The model under review builds one solid part; all positions refer to its coordinate system, in mm. A direction names the side the tool comes from. Give positions to 0.01 mm unless a question says otherwise; leave off trailing zeros. Loops run counter-clockwise (first coordinate to the right, second up) from the corner with the lowest first, then second, coordinate; pieces in that order, holes last. Notation, with made-up numbers: (9.5, -13.5) -> (17.5, -13.5) arc R15 ccw to (17.5, 9.5) -> close; hole circle Ø9 at (74.25, 60.5). An arc over 180 degrees is marked (long way). Write each question's results on one line, items separated by ' | '. Start each with the question number.
Q1. We need section C-C (x = -1). Write out the cut boundary in (y, z).
Q2. Wall thickness on L1, parallel to Z at x = 11, y = -2.7; L2, parallel to Y at x = 21.15, z = -9.9; L3, parallel to X at y = -1.25, z = -0.75: over which ranges is each line inside the solid? List them lowest first. Write a range as [from, to].
Q3. We need section A-A (y = -15.75). Write out the cut boundary in (x, z), plus the area to 3 significant figures.
Q4. Insertion check: pin 1 Ø15 at (x, y) = (2, -14.5) entering from +Z; pin 2 Ø8 at (x, z) = (-7, -0.5) entering from -Y; pin 3 Ø1.2 at (y, z) = (-1.5, -3) entering from +X; pin 4 Ø1.2 at (y, z) = (-2, -2) entering from -X. Each pin has a flat end and moves straight along its axis. Give the tip position at first contact, or say it passes through.
Q5. Mouldability with a two-part tool opening along Z and no side actions: class faces 4 (the face through (-23, -28, -10)), 5 (the face through (-12.5, -1.97, 0.07)), 6 (the face through (9.5, -1.97, 0.07)), 7 (the face through (2, -28, -8)) as released by +Z, released by -Z, zero draft, split by the parting line, or undercut.
Q6. We need section D-D (x = 11). Write out the cut boundary in (y, z).
Q7. Machinability: for faces 1 (the face through (6.707, -4.063, -9.972)), 2 (the face through (-19, -2, -2)), 3 (the face through (19, -2, -2)), which of the approach directions +Z, -Z, +X, -X, +Y, -Y give a long, thin tool a straight path to every point of the face, cutting with its end or side? Answer none if there is none.
Q8. We need section B-B (z = -9). Write out the cut boundary in (x, y).
from build123d import *

# Parameters (mm, degrees)
SKETCH_R             = 1.5
PAD_DEPTH            = 4
SKETCH001_R          = 0.5
PAD001_DEPTH         = 4
FILLET_R             = 4
CHAMFER_SIZE         = 4
BODY_PLACEMENT_ANGLE = 90


with BuildPart() as part:
    # Sketch → Pad (new body)
    with BuildSketch(Plane.XY):
        Polygon((-15, 4), (15, 4), (19, 0), (19, -8), (-19, -8), (-19, 0), align=None)
        with Locations((-11, 0)):
            Circle(SKETCH_R, mode=Mode.SUBTRACT)
        with Locations((11, 0)):
            Circle(SKETCH_R, mode=Mode.SUBTRACT)
    extrude(amount=PAD_DEPTH)

    # Sketch001 (on Face2 of Pad) → Pad001 (join)
    with BuildSketch(Plane.XZ.offset(8)):
        Polygon((-25, 30), (25, 30), (25, 0), (0, 0), (-25, 0), align=None)
        with Locations((-21.15, 24.5)):
            Circle(SKETCH001_R, mode=Mode.SUBTRACT)
        with Locations((-21.15, 7)):
            Circle(SKETCH001_R, mode=Mode.SUBTRACT)
        with Locations((21.15, 7)):
            Circle(SKETCH001_R, mode=Mode.SUBTRACT)
        with Locations((21.15, 24.5)):
            Circle(SKETCH001_R, mode=Mode.SUBTRACT)
        with BuildLine():
            ThreePointArc((-16.184193, 23.938422), (-21.85, 15.75), (-16.184193, 7.561578))
            Line((-16.184193, 7.561578), (-7.409917, 4.256721))
            ThreePointArc((-7.409917, 4.256721), (-6.716549, 4.064704), (-6, 4))
            Line((-6, 4), (0, 4))
            Line((6, 4), (0, 4))
            ThreePointArc((6, 4), (6.716549, 4.064704), (7.409917, 4.256721))
            Line((7.409917, 4.256721), (16.184193, 7.561578))
            ThreePointArc((16.184193, 7.561578), (21.85, 15.75), (16.184193, 23.938422))
            Line((16.184193, 23.938422), (7.409917, 27.243279))
            ThreePointArc((7.409917, 27.243279), (6.716549, 27.435296), (6, 27.5))
            Line((0, 27.5), (6, 27.5))
            Line((-6, 27.5), (0, 27.5))
            ThreePointArc((-6, 27.5), (-6.716549, 27.435296), (-7.409917, 27.243279))
            Line((-16.184193, 23.938422), (-7.409917, 27.243279))
        make_face(mode=Mode.SUBTRACT)
    extrude(amount=PAD001_DEPTH)

    # Fillet
    fillet_edges = [part.edges().sort_by_distance(p)[0] for p in [
        (19, -8, 2),
        (-19, -8, 2),
    ]]
    fillet(fillet_edges, radius=FILLET_R)

    # Chamfer
    chamfer_edges = [part.edges().sort_by_distance(p)[0] for p in [
        (-25, -10, 30),
        (25, -10, 30),
    ]]
    chamfer(chamfer_edges, length=CHAMFER_SIZE)


with BuildPart() as part_1:
    # Body placement: moved
    add(part.part.rotate(Axis((0, 0, 0), (1, 0, 0)), BODY_PLACEMENT_ANGLE))


solid = part_1.part
Output:
1) outline: (-30, -12) -> (-27.5, -12) -> (-27.5, -8) -> (-30, -8) -> close; (-4, -12) -> (0, -12) -> (0, 4) -> (-4, 4) -> close
2) L1: [-12, -1.5], [1.5, 4] | L2: [-29.85, -25], [-24, -19.18], [-12.32, -7.5], [-6.5, 0] | L3: [-19, -12.3], [-9.7, 9.7], [12.3, 19]
3) outline: (-25, -12) -> (-21.85, -12) -> (-21.85, -8) -> (-25, -8) -> close; (21.85, -12) -> (25, -12) -> (25, -8) -> (21.85, -8) -> close | area: 25.2 mm2
4) pin 1: through | pin 2: y = -4 | pin 3: x = 19 | pin 4: x = -19
5) face 4: zero draft | face 5: undercut | face 6: undercut | face 7: released by +Z
6) outline: (-30, -12) -> (-25.89, -12) -> (-25.89, -8) -> (-30, -8) -> close; (-5.61, -12) -> (0, -12) -> (0, -1.5) -> (-4, -1.5) -> (-4, -8) -> (-5.61, -8) -> close; (-4, 1.5) -> (0, 1.5) -> (0, 4) -> (-4, 4) -> close
7) face 1: +Z, -Z | face 2: +Z, -X, +Y, -Y | face 3: +Z, +X, +Y, -Y
8) outline: (-25, -26) -> (-21, -30) -> (21, -30) -> (25, -26) -> (25, 0) -> (-25, 0) -> close; hole circle Ø1 at (-21.15, -24.5); hole circle Ø1 at (-21.15, -7); hole (-16.18, -23.94) -> (-7.41, -27.24) arc R4 ccw to (-6, -27.5) -> (6, -27.5) arc R4 ccw to (7.41, -27.24) -> (16.18, -23.94) arc R8.75 ccw to (16.18, -7.56) -> (7.41, -4.26) arc R4 ccw to (6, -4) -> (-6, -4) arc R4 ccw to (-7.41, -4.26) -> (-16.18, -7.56) arc R8.75 ccw to start; hole circle Ø1 at (21.15, -24.5); hole circle Ø1 at (21.15, -7)
